Geometry: see drawing. Coordinates: mm, zero at the bounding-box minimum. Round coordinates to 2 decimals unless told otherwise and drop trailing zeros. Loops run counter-clockwise (first coordinate to the right, second up) from the corner with the lowest first, then second, coordinate; pieces in that order, holes last. Notation, with made-up numbers: (83.5, -38) - (99.5, -38) arc R20 cw to (99.5, -4) - close; hole circle Ø11 at (23.25, 52.5). An arc over 180 degrees is marked (long way). One line per question, with ' | ' between items. Start each with the question number.
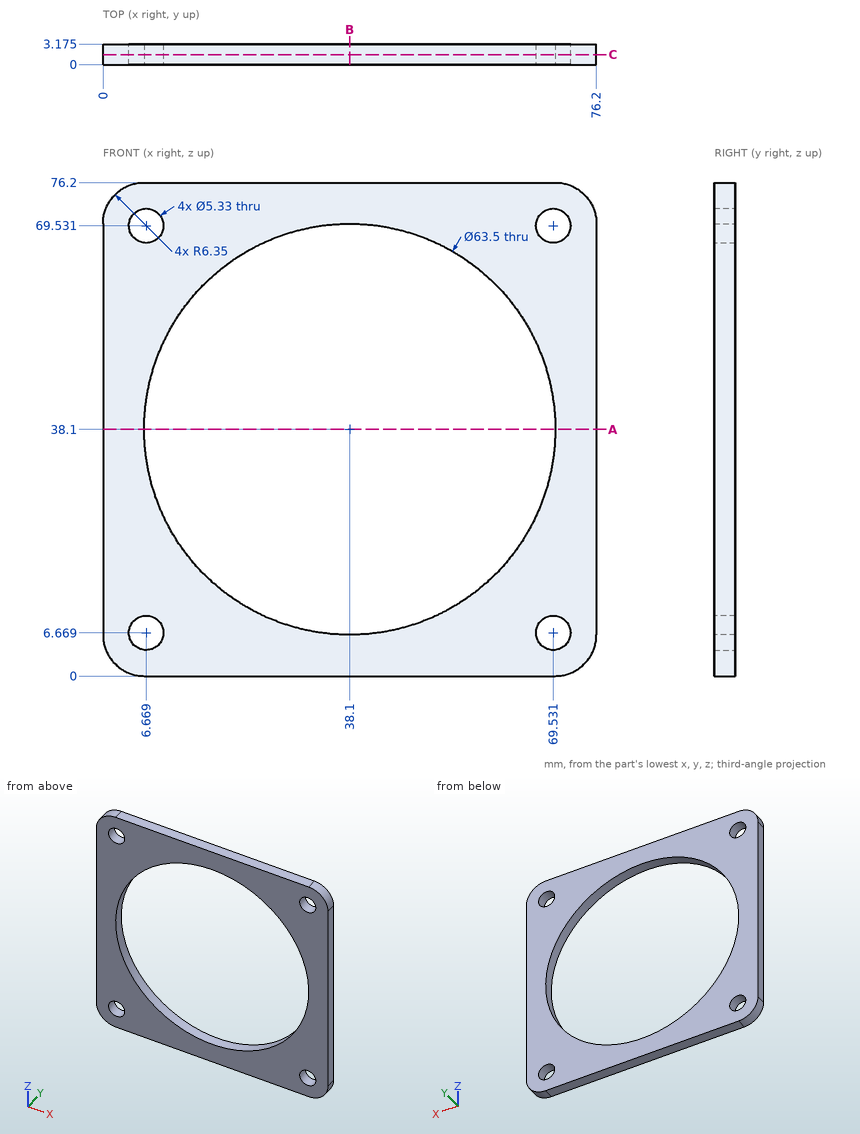
(1) Section B-B, the plane x = 38.1. Output: boundary loops of the cut face in (y, z) (3 decimals).
(2) Line query: line 1 along X through (y, z) = (0.4, 71) (1 decimal); line 2 along Z through (x, y) = (54.5, 1.75); line 3 along X through (y, z) = (1, 46). Output: solid intervals per line, ascending. Write a range as from..to.
(3) Pin query (flat end, axial travel): P1, Ø5, axis at x = 6.67, z = 6.67, coming from the -Y side. Return the tip coordinate at first contact, or that it passes through.
(4) Section C-C, the plane y = 1.55. Output: boundary loops of the cut face in (x, z) (3 decimals), plus the area to 3 significant figures.
(5) Section A-A, the plane z = 38.1. Output: boundary loops of the cut face in (x, y) (3 decimals).
Derived:
1) outline: (0, 0) - (3.175, 0) - (3.175, 6.35) - (0, 6.35) - close; (0, 69.85) - (3.175, 69.85) - (3.175, 76.2) - (0, 76.2) - close
2) line 1: x = 0.1..4.4, 8.9..67.3, 71.8..76.1 | line 2: z = 0..10.91, 65.29..76.2 | line 3: x = 0..7.35, 68.85..76.2
3) P1: passes through
4) outline: (0, 6.35) arc R6.35 ccw to (6.35, 0) - (69.85, 0) arc R6.35 ccw to (76.2, 6.35) - (76.2, 69.85) arc R6.35 ccw to (69.85, 76.2) - (6.35, 76.2) arc R6.35 ccw to (0, 69.85) - close; hole circle Ø5.33 at (6.669, 6.669); hole circle Ø5.33 at (6.669, 69.531); hole circle Ø63.5 at (38.1, 38.1); hole circle Ø5.33 at (69.531, 6.669); hole circle Ø5.33 at (69.531, 69.531) | area: 2,520 mm²
5) outline: (0, 0) - (6.35, 0) - (6.35, 3.175) - (0, 3.175) - close; (69.85, 0) - (76.2, 0) - (76.2, 3.175) - (69.85, 3.175) - close
